```python
from build123d import *
from OCP.BRepAlgoAPI import BRepAlgoAPI_Cut
from OCP.TopTools import TopTools_ListOfShape

# Parameters (mm, degrees)
SWEEP1_START       = -5
SWEEP1_DEPTH       = 10
SKETCH3_R          = 2.5
CUT_EXTRUDE1_DEPTH = 10
SKETCH6_R          = 2.5
CUT_EXTRUDE2_DEPTH = 2


with BuildPart() as part:
    # Sweep1: read off the stored shape, not the designer's step
    # Sweep1 outline → Sweep1 (new body)
    with BuildSketch(Plane.XY.offset(SWEEP1_START)):
        with BuildLine():
            Line((232.923534553, -10.606601718), (234.337748115, -9.192388155))
            Line((234.337748115, -9.192388155), (227.266680303, -2.121320344))
            add(Edge.make_bspline(
                [(220.973792806, 1.000000004), (220.996623613, 0.996738482), (221.019823203, 0.993424062), (221.32319859, 0.950076613), (221.626964068, 0.894672744), (222.202549229, 0.764511245), (222.487656849, 0.687861068), (223.332329716, 0.423928716), (223.881232147, 0.202580142), (225.463987163, -0.588990805), (226.43267267, -1.28731271), (227.266680303, -2.121320344)],
                knots=[-0.004264936, -0.004264936, -0.004264936, -0.004264936, 0, 0, 0.048942856, 0.048942856, 0.097885713, 0.097885713, 0.195771425, 0.195771425, 0.39154285, 0.39154285, 0.39154285, 0.39154285], degree=3))
            Line((220.973792806, 1.000000004), (-109.309697151, 0.999999892))
            ThreePointArc((-109.309697151, 0.999999892), (-113.470401554, 0.195974843), (-117.018410768, -2.121253679))
            Line((-117.018410768, -2.121253679), (-124.089413627, -9.192388155))
            Line((-124.089413627, -9.192388155), (-122.675200065, -10.606601718))
            Line((-122.675200065, -10.606601718), (-115.609189907, -3.540595572))
            ThreePointArc((-115.609189907, -3.540595572), (-112.70975362, -1.653770585), (-109.312780923, -1.000000132))
            Line((-109.312780923, -1.000000132), (220.829769992, -1))
            ThreePointArc((220.829769992, -1), (223.54434808, -1.865184594), (225.852466741, -3.535533906))
            Line((225.852466741, -3.535533906), (232.923534553, -10.606601718))
        make_face()
    extrude(amount=SWEEP1_DEPTH)


with BuildPart() as cut_extrude1_tool:
    # Sketch3 → Cut-Extrude1 (new body)
    with BuildSketch(Plane(origin=(-56.034299174, 56.034299174, 0), x_dir=(0, 0, -1), z_dir=(0.7071067811865286, -0.7071067811865666, 0))):
        with Locations(Location((0, -89.248043129, 0), (0, 0, 90))):
            Circle(SKETCH3_R)
    extrude(amount=-CUT_EXTRUDE1_DEPTH)


with BuildPart() as part_1:
    add(part.part)

    # Cut-Extrude1: cut by cut_extrude1_tool, with a tolerance
    cut_extrude1_stock = TopTools_ListOfShape()
    cut_extrude1_stock.Append(part_1.part.wrapped)
    cut_extrude1_tools = TopTools_ListOfShape()
    cut_extrude1_tools.Append(cut_extrude1_tool.part.wrapped)
    cut_extrude1_cut = BRepAlgoAPI_Cut()
    cut_extrude1_cut.SetArguments(cut_extrude1_stock)
    cut_extrude1_cut.SetTools(cut_extrude1_tools)
    cut_extrude1_cut.SetFuzzyValue(0.00001)
    cut_extrude1_cut.Build()
    add(Compound.cast(cut_extrude1_cut.Shape()).solids(), mode=Mode.REPLACE)

    # Sketch6 → Cut-Extrude2 (cut)
    with BuildSketch(Plane(origin=(111.158466417, 111.158466417, 0), x_dir=(0, 0, 1), z_dir=(-0.7071067811865477, -0.7071067811865475, 0))):
        with Locations(Location((0, -167.20181078, 0), (0, 0, 270))):
            Circle(SKETCH6_R)
    extrude(amount=-CUT_EXTRUDE2_DEPTH, mode=Mode.SUBTRACT)


solid = part_1.part
```
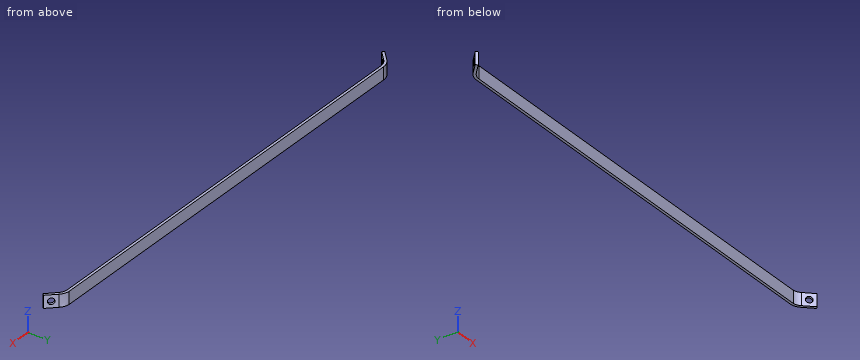
Can you work these out from the model? Positions are in its coordinate system, mm. Coordinates: 2 decimals unless noted, no trailing zeros. Loops run counter-clockwise (first coordinate to the right, second up) from the corner with the lowest first, then second, coordinate; pieces in that order, holes last. Notation, with made-up numbers: M 21,-6.75 L 26,-6.75 A11 ccw 26,13.25 Z; hole C -21,30 d4. An arc over 180 degrees is marked long. Put each result on its own line as item: value. Start each with the question number.
(1) I need wall thicknesses on probe 1 along Y at (x, z) = (164, -1); probe 2 along X at (y, z) = (-9, 0); probe 3 along X at (y, z) = (-8, -3.5). Which ranges of each line are inside material? Lowest first, please.
(2) Imagine slicing it at A-A on x = -24. List the corners of the cut face in (y, z) for me, and give its area (3 significant figures).
(3) Will these pins go through, and if not, where does the flat tip stop? pin 1 Ø1.5 at (y, z) = (-0.5, -1) entering from -X; pin 2 Ø1 at (y, z) = (-3.5, 0.5) entering from -X; pin 3 Ø5 at (y, z) = (-7.5, 4) entering from -X.
Worked answers:
1. probe 1: y = -1 to 1
1. probe 2: x = -123.9 to -121.07, 231.32 to 234.15
1. probe 3: x = -122.9 to -120.07, 230.32 to 233.15
2. outline: M -1,-5 L 1,-5 L 1,5 L -1,5 Z
2. area: 20.0 mm2
3. pin 1: stops at x = -116.01
3. pin 2: stops at x = -118.86
3. pin 3: stops at x = -124.09
